Input: part model. Units: mm. Frame: model coordinates. Face numbers are marked on the shaded views. A direction names the side the tool comes from. Give positions to 0.01 mm unless a question says otherwise; leave off trailing zeros. Loops run counter-clockwise (first coordinate to the right, second up) from the corner with the lowest first, then second, coordinate; pieces in that order, holes last. Notation, with made-up numbers: (-3.5, 7.25) - (31.5, 7.25) arc R30 cw to (31.5, 30.25) - close; hole circle Ø7 at (44.25, 5.5). An arc over 180 degrees is marked (long way). Answer as a JSON object with one key per item and string values.
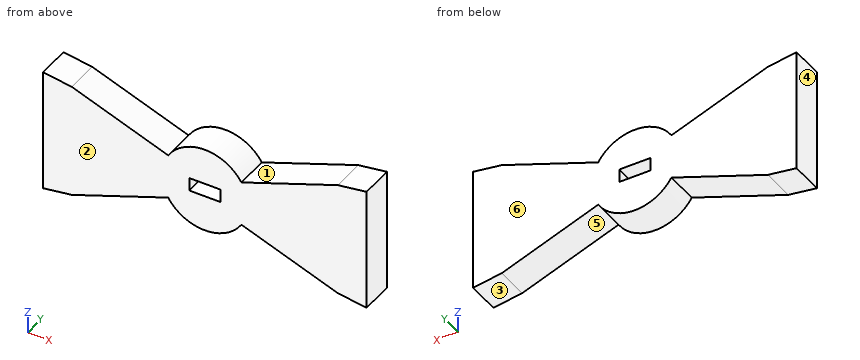
from build123d import *

# Parameters (mm, degrees)
BOSS_EXTRUDE3_DEPTH = 1.905
SKETCH2_W           = 1.778
SKETCH2_H           = 0.762
CUT_EXTRUDE1_DEPTH  = 2.54


with BuildPart() as part:
    # Sketch1 → Boss-Extrude3 (new body)
    with BuildSketch(Plane(origin=(0, 0, 0), x_dir=(1, 0, 0), z_dir=(0, 1, 0))):
        with BuildLine():
            Line((9.2654018, 3.543697889), (9.2654018, -3.543697889))
            Line((9.2654018, -3.543697889), (7.62, -3.302))
            Line((7.62, -3.302), (2.096490205, -1.291606846))
            ThreePointArc((2.096490205, -1.291606846), (0, -2.462421456), (-2.096490205, -1.291606846))
            Line((-2.096490205, -1.291606846), (-7.62, -3.302))
            Line((-7.62, -3.302), (-9.2654018, -3.543697889))
            Line((-9.2654018, -3.543697889), (-9.2654018, 3.543697889))
            Line((-9.2654018, 3.543697889), (-7.62, 3.302))
            Line((-7.62, 3.302), (-2.096490205, 1.291606846))
            ThreePointArc((-2.096490205, 1.291606846), (0, 2.462421456), (2.096490205, 1.291606846))
            Line((2.096490205, 1.291606846), (7.62, 3.302))
            Line((7.62, 3.302), (9.2654018, 3.543697889))
        make_face()
    extrude(amount=BOSS_EXTRUDE3_DEPTH)

    # Sketch2 → Cut-Extrude1 (cut)
    with BuildSketch(Plane(origin=(0, 1.905, 0), x_dir=(1, 0, 0), z_dir=(0, 1, 0))):
        Rectangle(SKETCH2_W, SKETCH2_H)
    extrude(amount=-CUT_EXTRUDE1_DEPTH, mode=Mode.SUBTRACT)


solid = part.part
Item 1: Cut plane C-C (z = 1.5). Return loops of the section in (x, y) (3 decimals).
Geometry check:
{"outline": "(-9.265, 0) - (-2.669, 0) - (-2.669, 1.905) - (-9.265, 1.905) - close; (-1.953, 0) - (1.953, 0) - (1.953, 1.905) - (-1.953, 1.905) - close; (2.669, 0) - (9.265, 0) - (9.265, 1.905) - (2.669, 1.905) - close"}
Item 2: Contact query for a flat-ended pin moving along its axis: P1, Ø0.5, axis at x = 0, y = 1, coming from the -Z side. Output: stop coordinate, or through.
Geometry check:
{"P1": "stops at z = -2.46"}
Item 3: Mould query, pull axis X, two halves, no side actions, for the marked faces 4, 5 and 6. Classes: released by +X, released by -X, zero draft, split by the parting line, or undercut.
Geometry check:
{"face 4": "released by -X", "face 5": "undercut", "face 6": "zero draft"}
Item 4: Material intervals for line 1 (Z direction, x = -4.75, y = 1.6); line 2 (Z direction, x = -4.5, y = 1.2), sorted ascending. Write a range as [from, to].
Geometry check:
{"line 1": "z = [-2.26, 2.26]", "line 2": "z = [-2.17, 2.17]"}
Item 5: Cut plane D-D (x = -0.25). Return loops of the section in (y, z) (3 decimals), then the cut area to 3 significant figures.
Geometry check:
{"outline": "(0, -2.45) - (1.905, -2.45) - (1.905, -0.381) - (0, -0.381) - close; (0, 0.381) - (1.905, 0.381) - (1.905, 2.45) - (0, 2.45) - close", "area": "7.88 mm2"}
Item 6: Cut plane A-A (y = 0.65). Return loops of the section in (x, z).
Geometry check:
{"outline": "(-9.27, -3.54) - (-7.62, -3.3) - (-2.1, -1.29) arc R2.46 ccw to (2.1, -1.29) - (7.62, -3.3) - (9.27, -3.54) - (9.27, 3.54) - (7.62, 3.3) - (2.1, 1.29) arc R2.46 ccw to (-2.1, 1.29) - (-7.62, 3.3) - (-9.27, 3.54) - close; hole (-0.89, -0.38) - (0.89, -0.38) - (0.89, 0.38) - (-0.89, 0.38) - close"}
Item 7: Access query for the marked faces 1, 2 and 3. Directions: +Z, -Z, +X, -X, +Y, -Y. A direction counts if a zero-diameter tool reaches every point of the face in a straight line with its end or side. Return the directions, or none.
Geometry check:
{"face 1": "+Z, +Y, -Y", "face 2": "+Z, -Z, +X, -X, -Y", "face 3": "-Z, +Y, -Y"}
Item 8: Cut plane B-B (z = -3). Return loops of the section in (x, y) (3 decimals).
Geometry check:
{"outline": "(-9.265, 0) - (-6.79, 0) - (-6.79, 1.905) - (-9.265, 1.905) - close; (6.79, 0) - (9.265, 0) - (9.265, 1.905) - (6.79, 1.905) - close"}
